Autodesk Inventor part; units mm, degrees
ref_plane "to_dummy_R_XY" through (0, 0, 0) normal (0, 0, 1) x (1, 0, 0)
ref_plane "to_dummy_R_YZ" through (0, 0, 0) normal (1, 0, 0) x (0, 1, 0)
ref_plane "to_dummy_R_ZX" through (0, 0, 0) normal (0, 1, 0) x (0, 0, 1)
sketch "Sketch_1" plane through (0, 0, 0) normal (1, 0, 0) x (0, 1, 0)
  line L0 (44.45, 0) -> (1.27, 0)
  arc A0 (1.27, 0) -> (0, -1.27) centre (1.27, -1.27) ccw
  line L1 (0, -1.27) -> (0, -25.4)
  line L2 (0, -25.4) -> (3.4163, -25.4)
  line L3 (3.4163, -25.4) -> (3.4163, -4.6863)
  arc A1 (4.6863, -3.4163) -> (3.4163, -4.6863) centre (4.6863, -4.6863) ccw
  line L4 (4.6863, -3.4163) -> (44.45, -3.4163)
  line L5 (44.45, -3.4163) -> (44.45, 0)
extrude "Extrusion1" add sketch "Sketch_1" along normal blind 38.1
sketch "Sketch_2" plane through (0, 0, 0) normal (0, 0, 1) x (1, 0, 0)
  line L0 (-38.1, -44.45) -> (57.15, -44.45)
  line L1 (57.15, -44.45) -> (57.15, 66.675)
  line L2 (57.15, 66.675) -> (-38.1, 66.675)
  line L3 (-38.1, 66.675) -> (-38.1, -44.45)
  line L4 (0, 0) -> (38.1, 0)
  line L5 (38.1, 0) -> (38.1, 6.35)
  line L6 (38.1, 6.35) -> (17.6579, 39.8829)
  arc A0 (17.6579, 39.8829) -> (0, 34.925) centre (9.525, 34.925) ccw
  line L7 (0, 34.925) -> (0, 0)
extrude "Extrusion2" cut sketch "Sketch_2" against normal blind 25.4
sketch "Sketch3" plane through (0, 1.27, 0) normal (0, 0, 1) x (1, 0, 0)
  point P0 (9.525, 33.655)
hole "Hole1" at (9.525, 34.925, 0) direction (0, 0, -1) diameter 9.5885 depth 3.4163
sketch "Sketch4" plane through (0, 0, -25.4) normal (0, -1, 0) x (1, 0, 0)
  point P0 (6.35, 9.525)
hole "Hole2" at (6.35, 0, -15.875) direction (0, 1, 0) diameter 6.7564 depth 3.4163
sketch "Sketch5" plane through (0, 0, -25.4) normal (0, -1, 0) x (1, 0, 0)
  point P0 (31.75, 9.525)
hole "Hole3" at (31.75, 0, -15.875) direction (0, 1, 0) diameter 6.7564 depth 3.4163
sketch "Sketch_6" plane through (0, 0, 0) normal (0, 1, 0) x (-1, 0, 0)
  line L0 (0, -19.2532) -> (0, -12.4968)
  line L1 (0, -12.4968) -> (-6.35, -12.4968)
  line L2 (-6.35, -12.4968) -> (-6.35, -19.2532)
  line L3 (-6.35, -19.2532) -> (0, -19.2532)
sketch "Sketch_7" plane through (0, 0, 0) normal (0, 1, 0) x (-1, 0, 0)
  line L0 (-31.75, -19.2532) -> (-31.75, -12.4968)
  line L1 (-31.75, -12.4968) -> (-38.1, -12.4968)
  line L2 (-38.1, -12.4968) -> (-38.1, -19.2532)
  line L3 (-38.1, -19.2532) -> (-31.75, -19.2532)
extrude "Extrusion3" cut sketch "Sketch_6" along normal blind 3.4163
extrude "Extrusion4" cut sketch "Sketch_7" along normal blind 3.4163
sketch "Sketch_8" plane through (0, 0, 0) normal (0, 1, 0) x (-1, 0, 0)
  line L0 (0, -38.1) -> (0, -24.13)
  arc A0 (-1.27, -25.4) -> (0, -24.13) centre (-1.27, -24.13) ccw
  line L1 (-1.27, -25.4) -> (-36.83, -25.4)
  arc A1 (-38.1, -24.13) -> (-36.83, -25.4) centre (-36.83, -24.13) ccw
  line L2 (-38.1, -24.13) -> (-38.1, -38.1)
  line L3 (-38.1, -38.1) -> (0, -38.1)
extrude "Extrusion5" cut sketch "Sketch_8" along normal blind 3.4163
ref_plane "to_dummy_R_XY" through (0, 0, 0) normal (0, 0, 1) x (1, 0, 0)
ref_plane "to_dummy_R_YZ" through (0, 0, 0) normal (1, 0, 0) x (0, 1, 0)
ref_plane "to_dummy_R_ZX" through (0, 0, 0) normal (0, 1, 0) x (0, 0, 1)
ref_plane "to_pin_R_XY" through (9.525, 34.925, 0) normal (0, 0, 1) x (1, 0, 0)
ref_plane "to_pin_R_YZ" through (9.525, 34.925, 0) normal (1, 0, 0) x (0, 1, 0)
ref_plane "to_pin_R_ZX" through (9.525, 34.925, 0) normal (0, 1, 0) x (0, 0, 1)
properties part number "D-14826" material "Steel"
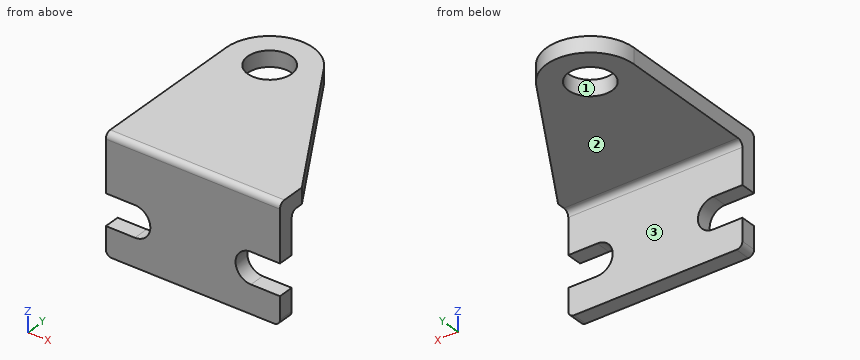
Here's how the part is built. I have some questions about the finished solid (model axes, mm). Face numbers are marked on the shaded views. Give positions to 0.01 mm unless a question says otherwise; leave off trailing zeros. Order: outer loops, then holes, each group sorted by start corner. A loop starts at its lowest first (then second) coordinate and runs counter-clockwise, first axis right, second up. Notation, with made-up numbers: (-19, 0) -> (33, 0) arc R28 ccw to (33, 20) -> close; hole circle Ø3 at (9, 71.5). An arc over 180 degrees is marked (long way). Use a Markdown table: item, result. Add a question column.
Item 1: I need wall thicknesses on line 1 (Y direction, x = 9.5, z = -2.5); line 2 (Y direction, x = 15, z = -14.75); line 3 (Z direction, x = 12, y = 24). Which ranges of each line are inside material? Lowest first, please.
Item 2: Imagine slicing it at A-A on y = 33.5. Please give me the cut outline in (x, z), plus the area to 3 significant figures.
Item 3: Imagine slicing it at B-B on x = 22.5. Please give me the cut outline in (y, z), plus the area to 3 significant figures.
Item 4: Imagine slicing it at D-D on x = 17. Please give me the cut outline in (y, z).
Item 5: If we mould it in two halves opening along Y, with no side actions, what happens to the marked faces 1, 2 and 3? For each: pulls with the +Y half, pulls with the -Y half, needs draft (parallel to the pull), parting line crosses it, or undercut.
Item 6: Imagine slicing it at C-C on z = -23.25. Please give me the cut outline in (x, y).
Item 7: Will these pins go through, and if not, where does the flat tip stop? pin 1 (12 mm diameter, centred on x = 12, y = 19.5, fed in from -Z); pin 2 (8 mm diameter, centred on x = 18, y = 9.5, fed in from +Z).
Data:
| question | item | result |
|---|---|---|
| 1 | line 1 | y = 0 to 30.13, 39.72 to 44.45 |
| 1 | line 2 | y = 0 to 3.42 |
| 1 | line 3 | z = -3.42 to 0 |
| 2 | outline | (0, -3.42) -> (4.95, -3.42) -> (4.95, 0) -> (0, 0) -> close; (14.1, -3.42) -> (21.55, -3.42) -> (21.55, 0) -> (14.1, 0) -> close |
| 2 | area | 42.3 mm² |
| 3 | outline | (0, -25.4) -> (3.42, -25.4) -> (3.42, -4.69) arc R1.27 cw to (4.69, -3.42) -> (31.94, -3.42) -> (31.94, 0) -> (1.27, 0) arc R1.27 ccw to (0, -1.27) -> close |
| 3 | area | 184 mm² |
| 4 | outline | (0, -25.4) -> (3.42, -25.4) -> (3.42, -4.69) arc R1.27 cw to (4.69, -3.42) -> (40.83, -3.42) -> (40.83, 0) -> (1.27, 0) arc R1.27 ccw to (0, -1.27) -> close |
| 5 | face 1 | undercut |
| 5 | face 2 | needs draft |
| 5 | face 3 | pulls with the +Y half |
| 6 | outline | (0, 0) -> (38.1, 0) -> (38.1, 3.42) -> (0, 3.42) -> close |
| 7 | pin 1 | stops at z = -3.42 |
| 7 | pin 2 | stops at z = 0 |
